Source: CAD feature listing. Evaluate the final solid. Frame: model axes, mm. Face numbers are marked on the shaded views. Coordinates: 2 decimals unless noted, no trailing zeros. Order: outer loops, then holes, each group sorted by start corner. A loop starts at its lowest first (then second) coordinate and runs counter-clockwise, first axis right, second up.
Item 1: Ray query, line 1 (Y direction, x = 0, z = -1); line 2 (X direction, y = 142, z = -0.5); line 3 (Y direction, x = -13, z = 12). Return the intervals inside material, ascending.
Item 2: Section D-D on x = 10. Return the cut outline in (y, z), then the cut area to 3 significant figures.
Item 3: Section A-A on x = 0. Return the cut outline in (y, z).
Item 4: Section B-B on y = 127. Return the cut outline in (x, z), then the cut area to 3 significant figures.
Item 5: Mould query, pull axis X, two halves, no side actions, for the marked faces 1, 2 and 3. Classes: released by +X, released by -X, zero draft, split by the parting line, or undercut.
Item 6: Contact query for flat-ended pins moving along their axis: P1, Ø12, axis at y = 173, z = 4, coming from the +X side; P2, Ø3, axis at y = 181.5, z = 7.5, coming from the +X side; P3, Ø2, axis at x = 11, z = -9.5, coming from the -Y side. Output: stop coordinate, or through.
Item 7: Section C-C on y = 32. Return the cut outline in (x, z), then the cut area to 3 significant figures.
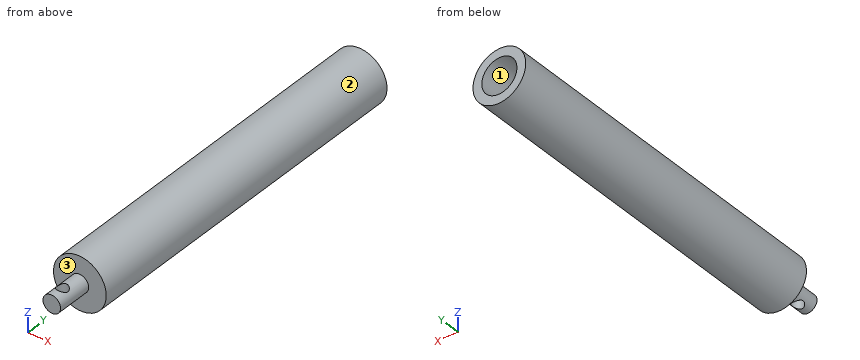
from build123d import *

# Parameters (mm, degrees)
SKETCH1_R               = 19.05
SKETCH1_R_2             = 6.35
BOSS_EXTRUDE1_DEPTH     = 254
SKETCH1_3_R             = 6.35
BOSS_EXTRUDE2_DEPTH     = 25.4
SKETCH2_R               = 12.7
CUT_EXTRUDE1_DEPTH      = 203.2
SKETCH3_R               = 3.96875
CUT_EXTRUDE2_DEPTH      = 256.424754086
CUT_EXTRUDE2_DEPTH_BACK = 256.424754086


with BuildPart() as part:
    # Sketch1 → Boss-Extrude1 (new body)
    with BuildSketch(Plane(origin=(0, 0, 0), x_dir=(1, 0, 0), z_dir=(0, 1, 0))):
        with Locations(Location((0, 0, 0), (0, 0, 270))):
            Circle(SKETCH1_R)
        Circle(SKETCH1_R_2, mode=Mode.SUBTRACT)
        Circle(SKETCH1_R_2)
    extrude(amount=BOSS_EXTRUDE1_DEPTH)

    # Sketch1_3 → Boss-Extrude2 (add)
    with BuildSketch(Plane(origin=(0, 0, 0), x_dir=(1, 0, 0), z_dir=(0, 1, 0))):
        with Locations(Location((0, 0, 0), (0, 0, 270))):
            Circle(SKETCH1_3_R)
    extrude(amount=-BOSS_EXTRUDE2_DEPTH)

    # Sketch2 → Cut-Extrude1 (cut)
    with BuildSketch(Plane(origin=(0, 254, 0), x_dir=(1, 0, 0), z_dir=(0, 1, 0))):
        with Locations(Location((0, 0, 0), (0, 0, 270))):
            Circle(SKETCH2_R)
    extrude(amount=-CUT_EXTRUDE1_DEPTH, mode=Mode.SUBTRACT)

    # Sketch3 → Cut-Extrude2 (cut, two sides)
    with BuildSketch(Plane.XY) as cut_extrude2_sk:
        with Locations((0, -15.875)):
            Circle(SKETCH3_R)
    extrude(amount=CUT_EXTRUDE2_DEPTH, mode=Mode.SUBTRACT)
    extrude(cut_extrude2_sk.sketch, amount=-CUT_EXTRUDE2_DEPTH_BACK, mode=Mode.SUBTRACT)


solid = part.part
Answer list:
1. line 1: y = -25.4 to -19.84, -11.91 to 50.8
1. line 2: x = -19.04 to -12.69, 12.69 to 19.04
1. line 3: y = 0 to 254
2. outline: (0, -16.21) - (254, -16.21) - (254, -7.83) - (50.8, -7.83) - (50.8, 7.83) - (254, 7.83) - (254, 16.21) - (0, 16.21) - close
2. area: 5,060 mm2
3. outline: (-25.4, -6.35) - (-19.84, -6.35) - (-19.84, 6.35) - (-25.4, 6.35) - close; (-11.91, -6.35) - (0, -6.35) - (0, -19.05) - (254, -19.05) - (254, -12.7) - (50.8, -12.7) - (50.8, 12.7) - (254, 12.7) - (254, 19.05) - (0, 19.05) - (0, 6.35) - (-11.91, 6.35) - close
4. outline: circle Ø38.1 at (0, 0); hole circle Ø25.4 at (0, 0)
4. area: 633 mm2
5. face 1: undercut
5. face 2: split by the parting line
5. face 3: zero draft
6. P1: stops at x = 19.05
6. P2: stops at x = 18.08
6. P3: stops at y = 0
7. outline: circle Ø38.1 at (0, 0)
7. area: 1,140 mm2
